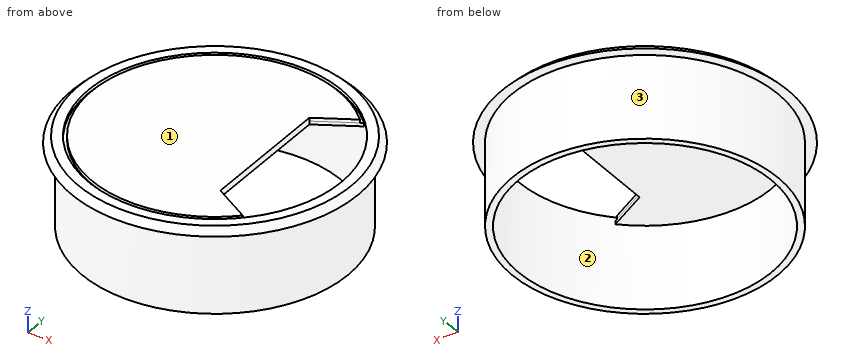
```python
from build123d import *

# Parameters (mm, degrees)
F3_DEPTH = 1
F5_DEPTH = 1


with BuildPart() as f1:
    # F0 (on Front) → F1 (revolve)
    with BuildSketch(Plane.XZ):
        Polygon((-38, -25), (-38, 2), (-41, 2), (-43, 0), (-40, 0), (-40, -25), align=None)
    revolve(axis=Axis((0, 0, -43.882875), (0, 0, -1)))

    # F2 (on Top) → F3 (join)
    with BuildSketch(Plane.XY):
        with BuildLine():
            Line((15, 20), (26.880754, 26.859357))
            ThreePointArc((26.880754, 26.859357), (-38, 0), (26.880754, -26.859357))
            Line((26.880754, -26.859357), (15, -20))
            Line((15, -20), (15, 20))
        make_face()
    extrude(amount=F3_DEPTH)

    # F4 (on face) → F5 (join, through all)
    with BuildSketch(Plane.XY.offset(1)):
        with BuildLine():
            Line((15, 20), (25.983406, 26.341272))
            ThreePointArc((25.983406, 26.341272), (-37, 0), (25.983406, -26.341272))
            Line((25.983406, -26.341272), (15, -20))
            Line((15, -20), (15, 20))
        make_face()
    extrude(amount=F5_DEPTH)


solid = f1.part
```
Part model, mm, in its own coordinate system. Face numbers are marked on the shaded views. Round coordinates to 2 decimals unless told otherwise and drop trailing zeros. Order: outer loops, then holes, each group sorted by start corner. A loop starts at its lowest first (then second) coordinate and runs counter-clockwise, first axis right, second up. Notation, with made-up numbers: M 53.5,58 L 85.5,58 A22 cw 85.5,87 Z; hole C -3.75,-37 d6. An arc over 180 degrees is marked long. Answer in a Markdown table with one row per item. Add a question column.
Q1. Pin check, flat tips, straight feed: pin 1 (4 mm diameter, centred on y = 29.5, z = -12, fed in from -X); pin 2 (12 mm diameter, centred on x = -9, y = 10.5, fed in from -Z); pin 3 (1.5 mm diameter, centred on y = 0, z = -16.5, fed in from +X). Stop position of each tip, or through.
Q2. Wall check: L1, parallel to Y at x = 0, z = -14.75; L2, parallel to Z at x = -1, y = -0.5; L3, parallel to X at y = 27, z = -3.75. Give the ranges that are in metal, low to high. Write a range as from..to.
Q3. Cut at C-C on z = -15.75. Give the cut face in (x, y), and give its area (3 significant figures).
Q4. Mould opens along Y. For the marked faces 1, 2 and 3 say: +Y half, -Y half, draft (parallel to the pull), parting line (faces both ways), or undercut.
Q5. Cut at A-A on y = 0. Give the cut face in (x, z).
Q6. Cut at B-B on x = 0. Give the cut face in (y, z).
Established:
| question | item | result |
|---|---|---|
| 1 | pin 1 | stops at x = -29.05 |
| 1 | pin 2 | stops at z = 0 |
| 1 | pin 3 | stops at x = 40 |
| 2 | L1 | y = -40..-38, 38..40 |
| 2 | L2 | z = 0..2 |
| 2 | L3 | x = -29.51..-26.74, 26.74..29.51 |
| 3 | outline | C 0,0 d80; hole C 0,0 d76 |
| 3 | area | 490 mm2 |
| 4 | face 1 | draft |
| 4 | face 2 | undercut |
| 4 | face 3 | parting line |
| 5 | outline | M -43,0 L -40,0 L -40,-25 L -38,-25 L -38,0 L 15,0 L 15,2 L -37,2 L -37,1 L -38,1 L -38,2 L -41,2 Z; M 38,-25 L 40,-25 L 40,0 L 43,0 L 41,2 L 38,2 Z |
| 6 | outline | M -43,0 L -40,0 L -40,-25 L -38,-25 L -38,0 L 38,0 L 38,-25 L 40,-25 L 40,0 L 43,0 L 41,2 L 38,2 L 38,1 L 37,1 L 37,2 L -37,2 L -37,1 L -38,1 L -38,2 L -41,2 Z |
